For this review, take the finished solid that the model builds, in its own axes (mm). Face numbers are marked on the shaded views. A direction names the side the tool comes from. Coordinates: 2 decimals unless noted, no trailing zeros. Order: outer loops, then holes, each group sorted by start corner. A loop starts at its lowest first (then second) coordinate and runs counter-clockwise, first axis right, second up. Notation, with made-up numbers: (39, 41) - (73, 41) arc R21 ccw to (73, 48) - close; hole circle Ø3 at (-35.75, -18.5). An arc over 180 degrees is marked (long way). One line per item, written item: value. Start each with the question number.
(1) Consider section B-B on z = 53.5. Write out the cut boundary in (x, y).
(2) For the marked faces 1, 2 and 3, list the 3-axis set-ups (+Z, -Z, +X, -X, +Y, -Y) from which the entire face can be reached by the end or side of a thin tool; tool diameter is ignored.
(3) Consider section C-C on z = 98. Write out the cut boundary in (x, y), then the cut area to 3 significant figures.
(4) Consider section A-A on x = 0. Count the separate pieces of the cut face and the enclosed holes in it, then the cut area to 3 significant figures.
(5) Clearance check with flat-ended pins moving along their axes: pin 1 (2 mm diameter, centred on x = 0, z = 10, fed in from -Y); pin 2 (5.5 mm diameter, centred on x = 23, z = 61, fed in from -Y); pin 3 (1 mm diameter, centred on x = -12.5, z = 23.5, fed in from -Y); pin 4 (0.8 mm diameter, centred on x = 22, y = 0.5, fed in from -Z). State where each tip first meets the part, or that it passes through.
(6) To check wall thickness, follow line 1 along X through (y, z) = (5.4, 28); line 2 along X through (y, z) = (2, 89.5). State the ranges of each line that lie inside material, in increasing order.
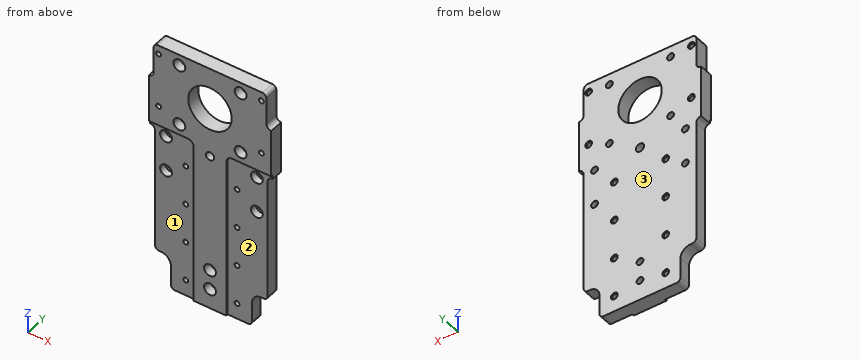
```python
from build123d import *

# Parameters (mm, degrees)
PLATE_MAIN_SKETCH_R             = 11
PLATE_MAIN_SKETCH_R_2           = 2.111650326
EXTRUDE_PLATE_MAIN_DEPTH        = 7
FILLET1_R                       = 2
M3X0_5_TAPPED_HOLE3_AT_2_COUNT  = 2
M3X0_5_TAPPED_HOLE3_AT_2_PITCH  = 27.5
M3X0_5_TAPPED_HOLE3_AT_3_COUNT  = 2
M3X0_5_TAPPED_HOLE3_AT_3_PITCH  = 58.823889705
M3X0_5_TAPPED_HOLE3_AT_4_COUNT  = 2
M3X0_5_TAPPED_HOLE3_AT_4_PITCH  = 66.206117542
M3X0_5_TAPPED_HOLE3_AT_5_COUNT  = 2
M3X0_5_TAPPED_HOLE3_AT_5_PITCH  = 83.20606949
M3X0_5_TAPPED_HOLE3_AT_6_COUNT  = 2
M3X0_5_TAPPED_HOLE3_AT_6_PITCH  = 101.307699609
M3X0_5_TAPPED_HOLE3_AT_7_COUNT  = 2
M3X0_5_TAPPED_HOLE3_AT_7_PITCH  = 120.013540903
M3X0_5_TAPPED_HOLE3_AT_8_COUNT  = 2
M3X0_5_TAPPED_HOLE3_AT_8_PITCH  = 114.242067558
M3X0_5_TAPPED_HOLE3_AT_9_COUNT  = 2
M3X0_5_TAPPED_HOLE3_AT_9_PITCH  = 94.399417371
M3X0_5_TAPPED_HOLE3_AT_10_COUNT = 2
M3X0_5_TAPPED_HOLE3_AT_10_PITCH = 74.640806534
M3X0_5_TAPPED_HOLE3_AT_11_COUNT = 2
M3X0_5_TAPPED_HOLE3_AT_11_PITCH = 55.056788864
M3X0_5_TAPPED_HOLE3_AT_12_COUNT = 2
M3X0_5_TAPPED_HOLE3_AT_12_PITCH = 52
CBORE_FOR_M3_SHCS1_AT_2_COUNT   = 2
CBORE_FOR_M3_SHCS1_AT_2_PITCH   = 31
CBORE_FOR_M3_SHCS1_AT_3_COUNT   = 2
CBORE_FOR_M3_SHCS1_AT_3_PITCH   = 43.840620434
CBORE_FOR_M3_SHCS1_AT_4_COUNT   = 2
CBORE_FOR_M3_SHCS1_AT_4_PITCH   = 31
CBORE_FOR_M3_SHCS1_AT_5_COUNT   = 2
CBORE_FOR_M3_SHCS1_AT_5_PITCH   = 42.172265768
CBORE_FOR_M3_SHCS1_AT_6_COUNT   = 2
CBORE_FOR_M3_SHCS1_AT_6_PITCH   = 56.608303278
CBORE_FOR_M3_SHCS1_AT_7_COUNT   = 2
CBORE_FOR_M3_SHCS1_AT_7_PITCH   = 70.86959856
CBORE_FOR_M3_SHCS1_AT_8_COUNT   = 2
CBORE_FOR_M3_SHCS1_AT_8_PITCH   = 59.970826241
CBORE_FOR_M3_SHCS1_AT_9_COUNT   = 2
CBORE_FOR_M3_SHCS1_AT_9_PITCH   = 101.688249075
CBORE_FOR_M3_SHCS1_AT_10_COUNT  = 2
CBORE_FOR_M3_SHCS1_AT_10_PITCH  = 111.581808553
CUT_RECESS_DEPTH                = 1


with BuildPart() as part:
    # Plate Main Sketch → Extrude Plate Main (new body)
    with BuildSketch(Plane(origin=(-158.085545862, 0, 24.679095537), x_dir=(-1, 0, 0), z_dir=(0, 1, 0))):
        with BuildLine():
            Line((-178.585545862, -24.679095537), (-137.585545862, -24.679095537))
            Line((-137.585545862, -24.679095537), (-137.585545862, -12.679095537))
            ThreePointArc((-137.585545862, -12.679095537), (-136.121079768, -9.143561631), (-132.585545862, -7.679095537))
            Line((-132.585545862, -7.679095537), (-129.585545862, -7.679095537))
            Line((-129.585545862, -7.679095537), (-129.585545862, 54.820904463))
            ThreePointArc((-129.585545862, 54.820904463), (-128.853312815, 56.588671416), (-127.085545862, 57.320904463))
            Line((-127.085545862, 57.320904463), (-127.085545862, 83.320904463))
            ThreePointArc((-127.085545862, 83.320904463), (-128.853312815, 84.05313751), (-129.585545862, 85.820904463))
            Line((-129.585545862, 85.820904463), (-129.585545862, 101.320904463))
            Line((-129.585545862, 101.320904463), (-186.585545862, 101.320904463))
            Line((-186.585545862, 101.320904463), (-186.585545862, 85.820904463))
            ThreePointArc((-186.585545862, 85.820904463), (-187.317778909, 84.05313751), (-189.085545862, 83.320904463))
            Line((-189.085545862, 83.320904463), (-189.085545862, 57.320904463))
            ThreePointArc((-189.085545862, 57.320904463), (-187.317778909, 56.588671416), (-186.585545862, 54.820904463))
            Line((-186.585545862, 54.820904463), (-186.585545862, -7.679095537))
            Line((-186.585545862, -7.679095537), (-183.585545862, -7.679095537))
            ThreePointArc((-183.585545862, -7.679095537), (-180.050011956, -9.143561631), (-178.585545862, -12.679095537))
            Line((-178.585545862, -12.679095537), (-178.585545862, -24.679095537))
        make_face()
        with Locations(Location((-158.085545862, 80.320904463, 0), (0, 0, 90))):
            Circle(PLATE_MAIN_SKETCH_R, mode=Mode.SUBTRACT)
        with Locations(Location((-158.085545862, 55.320904463, 0), (0, 0, 90))):
            Circle(PLATE_MAIN_SKETCH_R_2, mode=Mode.SUBTRACT)
    extrude(amount=EXTRUDE_PLATE_MAIN_DEPTH)

    # Fillet1
    fillet1_edges = [part.edges().sort_by_distance(p)[0] for p in [
        (28.5, 3.5, 126),
        (-28.5, 3.5, 126),
        (-28.5, 3.5, 17),
        (-20.5, 3.5, 0),
        (20.5, 3.5, 0),
        (28.5, 3.5, 17),
    ]]
    fillet(fillet1_edges, radius=FILLET1_R)

    # Sketch13 → M3x0.5 Tapped Hole3 (revolve, cut)
    with BuildSketch(Plane(origin=(26, 0, 121.5), x_dir=(0, 0, -1), z_dir=(1, 0, 0))):
        Polygon((0, 0), (0, 7), (1.725, 7), (1.25, 6.525), (1.25, 0), align=None)
    m3x0_5_tapped_hole3 = revolve(axis=Axis((26, -6.35, 121.5), (0, 1, 0)), mode=Mode.SUBTRACT)

    # M3x0.5 Tapped Hole3 at 2: M3x0.5 Tapped Hole3 ×2
    with Locations(*[(0, 0, -i * M3X0_5_TAPPED_HOLE3_AT_2_PITCH) for i in range(1, M3X0_5_TAPPED_HOLE3_AT_2_COUNT)]):
        add(m3x0_5_tapped_hole3, mode=Mode.SUBTRACT)

    # M3x0.5 Tapped Hole3 at 3: M3x0.5 Tapped Hole3 ×2
    with Locations(*[Vector(-0.8839945855497452, 0, -0.46749713658880765) * (i * M3X0_5_TAPPED_HOLE3_AT_3_PITCH) for i in range(1, M3X0_5_TAPPED_HOLE3_AT_3_COUNT)]):
        add(m3x0_5_tapped_hole3, mode=Mode.SUBTRACT)

    # M3x0.5 Tapped Hole3 at 4: M3x0.5 Tapped Hole3 ×2
    with Locations(*[Vector(-0.5890694311623529, 0, -0.8080824247996377) * (i * M3X0_5_TAPPED_HOLE3_AT_4_PITCH) for i in range(1, M3X0_5_TAPPED_HOLE3_AT_4_COUNT)]):
        add(m3x0_5_tapped_hole3, mode=Mode.SUBTRACT)

    # M3x0.5 Tapped Hole3 at 5: M3x0.5 Tapped Hole3 ×2
    with Locations(*[Vector(-0.46871580689935055, 0, -0.8833490206949294) * (i * M3X0_5_TAPPED_HOLE3_AT_5_PITCH) for i in range(1, M3X0_5_TAPPED_HOLE3_AT_5_COUNT)]):
        add(m3x0_5_tapped_hole3, mode=Mode.SUBTRACT)

    # M3x0.5 Tapped Hole3 at 6: M3x0.5 Tapped Hole3 ×2
    with Locations(*[Vector(-0.38496580369162126, 0, -0.9229308370555532) * (i * M3X0_5_TAPPED_HOLE3_AT_6_PITCH) for i in range(1, M3X0_5_TAPPED_HOLE3_AT_6_COUNT)]):
        add(m3x0_5_tapped_hole3, mode=Mode.SUBTRACT)

    # M3x0.5 Tapped Hole3 at 7: M3x0.5 Tapped Hole3 ×2
    with Locations(*[Vector(-0.32496333085967716, 0, -0.9457266167326497) * (i * M3X0_5_TAPPED_HOLE3_AT_7_PITCH) for i in range(1, M3X0_5_TAPPED_HOLE3_AT_7_COUNT)]):
        add(m3x0_5_tapped_hole3, mode=Mode.SUBTRACT)

    # M3x0.5 Tapped Hole3 at 8: M3x0.5 Tapped Hole3 ×2
    with Locations(*[Vector(-0.113793458730633, 0, -0.993504428148219) * (i * M3X0_5_TAPPED_HOLE3_AT_8_PITCH) for i in range(1, M3X0_5_TAPPED_HOLE3_AT_8_COUNT)]):
        add(m3x0_5_tapped_hole3, mode=Mode.SUBTRACT)

    # M3x0.5 Tapped Hole3 at 9: M3x0.5 Tapped Hole3 ×2
    with Locations(*[Vector(-0.13771271435815216, 0, -0.9904722148067102) * (i * M3X0_5_TAPPED_HOLE3_AT_9_PITCH) for i in range(1, M3X0_5_TAPPED_HOLE3_AT_9_COUNT)]):
        add(m3x0_5_tapped_hole3, mode=Mode.SUBTRACT)

    # M3x0.5 Tapped Hole3 at 10: M3x0.5 Tapped Hole3 ×2
    with Locations(*[Vector(-0.17416746420246676, 0, -0.9847160476062541) * (i * M3X0_5_TAPPED_HOLE3_AT_10_PITCH) for i in range(1, M3X0_5_TAPPED_HOLE3_AT_10_COUNT)]):
        add(m3x0_5_tapped_hole3, mode=Mode.SUBTRACT)

    # M3x0.5 Tapped Hole3 at 11: M3x0.5 Tapped Hole3 ×2
    with Locations(*[Vector(-0.23611983677697992, 0, -0.9717239436591096) * (i * M3X0_5_TAPPED_HOLE3_AT_11_PITCH) for i in range(1, M3X0_5_TAPPED_HOLE3_AT_11_COUNT)]):
        add(m3x0_5_tapped_hole3, mode=Mode.SUBTRACT)

    # M3x0.5 Tapped Hole3 at 12: M3x0.5 Tapped Hole3 ×2
    with Locations(*[(-i * M3X0_5_TAPPED_HOLE3_AT_12_PITCH, 0, 0) for i in range(1, M3X0_5_TAPPED_HOLE3_AT_12_COUNT)]):
        add(m3x0_5_tapped_hole3, mode=Mode.SUBTRACT)

    # Sketch5 → CBORE for M3 SHCS1 (revolve, cut)
    with BuildSketch(Plane(origin=(-15.5, 0, 120.5), x_dir=(0, 0, -1), z_dir=(1, 0, 0))):
        Polygon((0, 0), (0, 7), (1.725, 7), (1.7, 6.975), (1.7, 4.5), (3, 4.5), (3, 0), align=None)
    cbore_for_m3_shcs1 = revolve(axis=Axis((-15.5, -6.35, 120.5), (0, 1, 0)), mode=Mode.SUBTRACT)

    # CBORE for M3 SHCS1 at 2: CBORE for M3 SHCS1 ×2
    with Locations(*[(i * CBORE_FOR_M3_SHCS1_AT_2_PITCH, 0, 0) for i in range(1, CBORE_FOR_M3_SHCS1_AT_2_COUNT)]):
        add(cbore_for_m3_shcs1, mode=Mode.SUBTRACT)

    # CBORE for M3 SHCS1 at 3: CBORE for M3 SHCS1 ×2
    with Locations(*[Vector(0.7071067811865479, 0, -0.7071067811865472) * (i * CBORE_FOR_M3_SHCS1_AT_3_PITCH) for i in range(1, CBORE_FOR_M3_SHCS1_AT_3_COUNT)]):
        add(cbore_for_m3_shcs1, mode=Mode.SUBTRACT)

    # CBORE for M3 SHCS1 at 4: CBORE for M3 SHCS1 ×2
    with Locations(*[(0, 0, -i * CBORE_FOR_M3_SHCS1_AT_4_PITCH) for i in range(1, CBORE_FOR_M3_SHCS1_AT_4_COUNT)]):
        add(cbore_for_m3_shcs1, mode=Mode.SUBTRACT)

    # CBORE for M3 SHCS1 at 5: CBORE for M3 SHCS1 ×2
    with Locations(*[Vector(-0.1778419978967634, 0, -0.9840590550287557) * (i * CBORE_FOR_M3_SHCS1_AT_5_PITCH) for i in range(1, CBORE_FOR_M3_SHCS1_AT_5_COUNT)]):
        add(cbore_for_m3_shcs1, mode=Mode.SUBTRACT)

    # CBORE for M3 SHCS1 at 6: CBORE for M3 SHCS1 ×2
    with Locations(*[Vector(0.6801122409730789, 0, -0.7331080000099417) * (i * CBORE_FOR_M3_SHCS1_AT_6_PITCH) for i in range(1, CBORE_FOR_M3_SHCS1_AT_6_COUNT)]):
        add(cbore_for_m3_shcs1, mode=Mode.SUBTRACT)

    # CBORE for M3 SHCS1 at 7: CBORE for M3 SHCS1 ×2
    with Locations(*[Vector(0.5432512781572745, 0, -0.8395701571521512) * (i * CBORE_FOR_M3_SHCS1_AT_7_PITCH) for i in range(1, CBORE_FOR_M3_SHCS1_AT_7_COUNT)]):
        add(cbore_for_m3_shcs1, mode=Mode.SUBTRACT)

    # CBORE for M3 SHCS1 at 8: CBORE for M3 SHCS1 ×2
    with Locations(*[Vector(-0.12506080823181873, 0, -0.9921490786390946) * (i * CBORE_FOR_M3_SHCS1_AT_8_PITCH) for i in range(1, CBORE_FOR_M3_SHCS1_AT_8_COUNT)]):
        add(cbore_for_m3_shcs1, mode=Mode.SUBTRACT)

    # CBORE for M3 SHCS1 at 9: CBORE for M3 SHCS1 ×2
    with Locations(*[Vector(0.15242665834989907, 0, -0.9883147847848291) * (i * CBORE_FOR_M3_SHCS1_AT_9_PITCH) for i in range(1, CBORE_FOR_M3_SHCS1_AT_9_COUNT)]):
        add(cbore_for_m3_shcs1, mode=Mode.SUBTRACT)

    # CBORE for M3 SHCS1 at 10: CBORE for M3 SHCS1 ×2
    with Locations(*[Vector(0.13891153227375555, 0, -0.9903047945967733) * (i * CBORE_FOR_M3_SHCS1_AT_10_PITCH) for i in range(1, CBORE_FOR_M3_SHCS1_AT_10_COUNT)]):
        add(cbore_for_m3_shcs1, mode=Mode.SUBTRACT)

    # Reccess Sketch → Cut Recess (cut)
    with BuildSketch(Plane(origin=(0, 0, 0), x_dir=(1, 0, 0), z_dir=(0, 1, 0))):
        with BuildLine():
            Line((-8.25, 0), (-8.25, -81))
            ThreePointArc((-8.25, -81), (-9.128679656, -83.121320344), (-11.25, -84))
            Line((-11.25, -84), (-31, -84))
            Line((-31, -84), (-31, 0))
            Line((-31, 0), (-8.25, 0))
        make_face()
        with BuildLine():
            Line((31, 0), (8.25, 0))
            Line((8.25, 0), (8.25, -81))
            ThreePointArc((8.25, -81), (9.128679656, -83.121320344), (11.25, -84))
            Line((11.25, -84), (31, -84))
            Line((31, -84), (31, 0))
        make_face()
    extrude(amount=CUT_RECESS_DEPTH, mode=Mode.SUBTRACT)


solid = part.part
```
Geometry check:
1. outline: (-28.5, 1) - (-8.25, 1) - (-8.25, 0) - (8.25, 0) - (8.25, 1) - (28.5, 1) - (28.5, 7) - (-28.5, 7) - close
2. face 1: -Z, -X, -Y
2. face 2: -Z, +X, -Y
2. face 3: +Z, -Z, +X, -X, +Y
3. outline: (-31, 0) - (-8.49, 0) - (-8.49, 7) - (-31, 7) - close; (8.49, 0) - (31, 0) - (31, 7) - (8.49, 7) - close
3. area: 315 mm^2
4. separate pieces: 5
4. enclosed holes: 0
4. area: 627 mm^2
5. pin 1: passes through
5. pin 2: stops at y = 4.5
5. pin 3: stops at y = 1
5. pin 4: stops at z = 84
6. line 1: x = -28.5 to -14.25, -11.75 to 11.75, 14.25 to 28.5
6. line 2: x = -31 to -18.5, -12.5 to 12.5, 18.5 to 31
